The model under review builds one solid part; all positions refer to its coordinate system, in mm. Round coordinates to 2 decimals unless told otherwise and drop trailing zeros. Write each loop counter-clockwise with the first axis right and the second up, starting at its lowest first coordinate (ties: lowest second). Pieces come first, ordered by that corner, then holes. Notation, with made-up numbers: (-39, 21.5) -> (-32, 21.5) arc R18 cw to (-32, 53.5) -> close; hole circle Ø11 at (39.25, 25). An arc over 180 degrees is marked (long way). Answer in a Markdown table with one row per item. Add a question column.
```python
from build123d import *

# Parameters (mm, degrees)
F0_R     = 40
F1_DEPTH = 100


with BuildPart() as f1:
    # F0 (on Top) → F1 (new body)
    with BuildSketch(Plane.XY):
        with BuildLine():
            ThreePointArc((-849.0953685383, -259.2832277711), (-739.9313653682, -149.5470002399), (-700, 0))
            Line((-700, 0), (-850, 0))
            ThreePointArc((-850, 0), (-1000, -150), (-1150, 0))
            Line((-1150, 0), (-1300, 0))
            ThreePointArc((-1300, 0), (-1153.2850393406, -257.8831066867), (-856.6420219043, -263.5308143582))
            ThreePointArc((-856.6420219043, -263.5308143582), (-852.8801904642, -261.3865975578), (-849.0953685383, -259.2832277711))
        make_face()
        with BuildLine():
            ThreePointArc((-849.0953685383, 259.2832277711), (-739.9313653682, 149.5470002399), (-700, 0))
            Line((-700, 0), (-500, 0))
            ThreePointArc((-500, 0), (-472.4467242206, 163.6890123778), (-392.8236289072, 309.3373507551))
            ThreePointArc((-392.8236289072, 309.3373507551), (-613.0653910459, 212.3510174227), (-849.0953685383, 259.2832277711))
        make_face()
        with BuildLine():
            Line((-850, 0), (-700, 0))
            ThreePointArc((-700, 0), (-739.9313653682, 149.5470002399), (-849.0953685383, 259.2832277711))
            ThreePointArc((-849.0953685383, 259.2832277711), (-852.8801904642, 261.3865975578), (-856.6420219043, 263.5308143582))
            ThreePointArc((-856.6420219043, 263.5308143582), (-1153.2850393406, 257.8831066867), (-1300, 0))
            Line((-1300, 0), (-1150, 0))
            ThreePointArc((-1150, 0), (-1000, 150), (-850, 0))
        make_face()
        with BuildLine():
            Line((-500, 0), (-700, 0))
            ThreePointArc((-700, 0), (-739.9313653682, -149.5470002399), (-849.0953685383, -259.2832277711))
            ThreePointArc((-849.0953685383, -259.2832277711), (-613.0653910459, -212.3510174227), (-392.8236289072, -309.3373507551))
            ThreePointArc((-392.8236289072, -309.3373507551), (-472.4467242206, -163.6890123778), (-500, 0))
        make_face()
        with BuildLine():
            ThreePointArc((-392.8236289072, 309.3373507551), (-472.4467242206, 163.6890123778), (-500, 0))
            Line((-500, 0), (-20, 0))
            ThreePointArc((-20, 0), (36.5716696241, 147.2792613729), (177.1925530051, 218.8145798652))
            Line((177.1925530051, 218.8145798652), (314.6601955249, 388.5729807285))
            ThreePointArc((314.6601955249, 388.5729807285), (187.4065310938, 463.5502045123), (43.7997133909, 498.0778906023))
            ThreePointArc((43.7997133909, 498.0778906023), (-198.3939798634, 458.9551489568), (-392.8236289072, 309.3373507551))
        make_face()
        with BuildLine():
            ThreePointArc((-406.6148611623, 92.9051428836), (-169.1586966122, 377.4272459242), (200, 344.8678553104))
            ThreePointArc((200, 344.8678553104), (221.7006400578, 309.2991411686), (200, 273.7304270267))
            ThreePointArc((200, 273.7304270267), (37.9889182283, 215.8833684246), (-43.9509044765, 64.6228704059))
            ThreePointArc((-43.9509044765, 64.6228704059), (-56.0926702606, 37.1503028891), (-83.9313566685, 25.8732473601))
            Line((-83.9313566685, 25.8732473601), (-377.1313636694, 25.8732473601))
            ThreePointArc((-377.1313636694, 25.8732473601), (-413.7460862611, 49.7685247754), (-406.6148611623, 92.9051428836))
        make_face(mode=Mode.SUBTRACT)
        with BuildLine():
            Line((-20, 0), (-500, 0))
            ThreePointArc((-500, 0), (-472.4467242206, -163.6890123778), (-392.8236289072, -309.3373507551))
            ThreePointArc((-392.8236289072, -309.3373507551), (163.6890123778, -472.4467242206), (500, 0))
            ThreePointArc((500, 0), (498.8554636471, 33.8116309782), (495.4270944424, 67.4684673932))
            ThreePointArc((495.4270944424, 67.4684673932), (495.2295651607, 68.8764953304), (495.0353730255, 70.2849873978))
            ThreePointArc((495.0353730255, 70.2849873978), (435.0040690697, 246.5186806164), (314.6601955249, 388.5729807285))
            Line((314.6601955249, 388.5729807285), (177.1925530051, 218.8145798652))
            ThreePointArc((177.1925530051, 218.8145798652), (347.2792613729, 163.4283303759), (420, 0))
            ThreePointArc((420, 0), (200, -220), (-20, 0))
        make_face()
        with BuildLine():
            ThreePointArc((-406.6148611623, -102.8346635677), (-413.7460862611, -59.6980454595), (-377.1313636694, -35.8027680442))
            Line((-377.1313636694, -35.8027680442), (-83.9313566685, -35.8027680442))
            ThreePointArc((-83.9313566685, -35.8027680442), (-55.2084121975, -47.9640816364), (-43.9509044765, -77.0531449985))
            ThreePointArc((-43.9509044765, -77.0531449985), (41.5727461521, -229.7491196269), (200, -304.1208933235))
            ThreePointArc((200, -304.1208933235), (225.7915227703, -357.1958613892), (182.8680932522, -397.6894915104))
            ThreePointArc((182.8680932522, -397.6894915104), (-165.7061110263, -357.8861419627), (-406.6148611623, -102.8346635677))
        make_face(mode=Mode.SUBTRACT)
        with BuildLine():
            ThreePointArc((177.1925530051, 218.8145798652), (36.5716696241, 147.2792613729), (-20, 0))
            Line((-20, 0), (0, 0))
            Line((0, 0), (89.7600051949, 110.8443751857))
            ThreePointArc((89.7600051949, 110.8443751857), (94.1057606724, 154.5806536289), (135.9827631274, 167.9247275238))
            Line((135.9827631274, 167.9247275238), (177.1925530051, 218.8145798652))
        make_face()
        with BuildLine():
            Line((0, 0), (-20, 0))
            ThreePointArc((-20, 0), (200, -220), (420, 0))
            ThreePointArc((420, 0), (347.2792613729, 163.4283303759), (177.1925530051, 218.8145798652))
            Line((177.1925530051, 218.8145798652), (135.9827631274, 167.9247275238))
            ThreePointArc((135.9827631274, 167.9247275238), (157.0635818103, 153.5775860217), (165.1915991306, 129.4078379869))
            ThreePointArc((165.1915991306, 129.4078379869), (134.750266469, 90.5667273088), (89.7600051949, 110.8443751857))
            Line((89.7600051949, 110.8443751857), (0, 0))
        make_face()
        with Locations((125.1915991306, -127.0277351141)):
            Circle(F0_R, mode=Mode.SUBTRACT)
        with Locations((277.0611941814, -127.0277351141)):
            Circle(F0_R, mode=Mode.SUBTRACT)
        with BuildLine():
            ThreePointArc((100, 0), (60, -40), (20, 0))
            ThreePointArc((20, 0), (60, 40), (100, 0))
        make_face(mode=Mode.SUBTRACT)
        with Locations((340, 0)):
            Circle(F0_R, mode=Mode.SUBTRACT)
        with Locations((277.0611941814, 129.4078379869)):
            Circle(F0_R, mode=Mode.SUBTRACT)
        with BuildLine():
            ThreePointArc((508.4647709692, 972.9408629012), (347.8579835974, 665.3239807328), (43.7997133909, 498.0778906023))
            ThreePointArc((43.7997133909, 498.0778906023), (187.4065310938, 463.5502045123), (314.6601955249, 388.5729807285))
            Line((314.6601955249, 388.5729807285), (597.8543714973, 738.2886633841))
            ThreePointArc((597.8543714973, 738.2886633841), (521.5619679737, 843.5778116935), (508.4647709692, 972.9408629012))
        make_face()
        with BuildLine():
            Line((597.8543714973, 738.2886633841), (314.6601955249, 388.5729807285))
            ThreePointArc((314.6601955249, 388.5729807285), (435.0040690697, 246.5186806164), (495.0353730255, 70.2849873978))
            ThreePointArc((495.0353730255, 70.2849873978), (564.4809221518, 441.9510892686), (842.4187636125, 698.2886242833))
            ThreePointArc((842.4187636125, 698.2886242833), (714.8315735034, 685.8533594049), (597.8543714973, 738.2886633841))
        make_face()
        with BuildLine():
            ThreePointArc((1005.1844692598, 932.5751537484), (775.4338572426, 1181.7537288433), (508.4647709692, 972.9408629012))
            ThreePointArc((508.4647709692, 972.9408629012), (521.5619679737, 843.5778116935), (597.8543714973, 738.2886633841))
            ThreePointArc((597.8543714973, 738.2886633841), (714.8315735034, 685.8533594049), (842.4187636125, 698.2886242833))
            ThreePointArc((842.4187636125, 698.2886242833), (853.4019929681, 703.1204808996), (864.4796509854, 707.7317343393))
            ThreePointArc((864.4796509854, 707.7317343393), (967.1087428004, 799.9550109182), (1005.1844692598, 932.5751537484))
        make_face()
        with BuildLine():
            ThreePointArc((855.1844692598, 932.5751537484), (798.2355789406, 842.3166253134), (692.2524301548, 854.8605576027))
            ThreePointArc((692.2524301548, 854.8605576027), (677.4698731141, 995.5071928533), (818.1165083648, 1010.2897498941))
            ThreePointArc((818.1165083648, 1010.2897498941), (845.4429976948, 975.6262634292), (855.1844692598, 932.5751537484))
        make_face(mode=Mode.SUBTRACT)
    extrude(amount=F1_DEPTH)


solid = f1.part
```
1. Mouldability with a two-part tool opening along X and no side actions: class faces 1 (the cylindrical face through (268.39, 90.36, 49.3)), 2 (the cylindrical face through (-850.145, 6.595, 49.3)), 3 (the flat face through (103, 221, 0)) as pulls with the +X half, pulls with the -X half, needs draft (parallel to the pull), parting line crosses it, or undercut.
2. Add section A-A on x = -1000. Write out the cut boundary in (y, z).
3. Insertion check: pin 1 Ø3 at (y, z) = (408.5, 76.5) entering from -X; pin 2 Ø3 at (x, z) = (-807.5, 52.5) entering from -Y; pin 3 Ø12 at (x, z) = (249.5, 37) entering from -Y. Each pin has a flat end and moves straight along its axis. Give the tip position at first contact, or say it passes through.
4. For L1, parallel to X at y = -267.5, z = 41.5; L2, parallel to Y at x = -292.5, z = 28; L3, parallel to Y at x = 60, z = 24, list the stretches that pass through material, from the lowest coordinate up.
5. Add section B-B on z = 49. State how many separate pieces and enclosed holes the cut face has, plus the area to 3 significant figures.
6. Add section C-C on y = 737.5. Write out the cut boundary in (x, z), plus the area to 3 significant figures.
7. Add section D-D on x = -695. Write out the cut boundary in (y, z), plus the area to 3 significant figures.
Filled in:
| question | item | result |
|---|---|---|
| 1 | face 1 | undercut |
| 1 | face 2 | undercut |
| 1 | face 3 | needs draft |
| 2 | outline | (-300, 0) -> (-150, 0) -> (-150, 100) -> (-300, 100) -> close; (150, 0) -> (300, 0) -> (300, 100) -> (150, 100) -> close |
| 3 | pin 1 | x = -290.43 |
| 3 | pin 2 | y = -240.1 |
| 3 | pin 3 | y = -436.7 |
| 4 | L1 | -1135.81 to -864.19, -450 to -293.09, 92.41 to 422.43 |
| 4 | L2 | -405.52 to -268.07, -35.8 to 25.87, 296.81 to 405.52 |
| 4 | L3 | -496.39 to -411.91, -245.5 to -40, 40 to 232.65, 400.79 to 501.76 |
| 5 | separate pieces | 1 |
| 5 | enclosed holes | 10 |
| 5 | area | 1,130,000 mm² |
| 6 | outline | (408.17, 0) -> (911.54, 0) -> (911.54, 100) -> (408.17, 100) -> close |
| 6 | area | 50,300 mm² |
| 7 | outline | (-211.8, 0) -> (211.8, 0) -> (211.8, 100) -> (-211.8, 100) -> close |
| 7 | area | 42,400 mm² |
